```python
from build123d import *

# Parameters (mm, degrees)
BOSS_EXTRUDE1_DEPTH       = 51
BOSS_EXTRUDE3_DEPTH       = 51
SKETCH2_5_R               = 4.5
BOSS_EXTRUDE4_DEPTH       = 9
CUT_EXTRUDE2_REACH        = 105.296
SKETCH3_R                 = 4.5
CUT_EXTRUDE3_REACH        = 105.296
BOSS_EXTRUDE5_REACH       = 105.296
SKETCH4_R                 = 8
F_6_0MM_DOWEL_HOLE1_D     = 6
F_6_0MM_DOWEL_HOLE1_DEPTH = 13
F_6_0MM_DOWEL_HOLE1_TIP   = 1.802581857


with BuildPart() as part:
    # Sketch2 → Boss-Extrude1 (new body)
    with BuildSketch(Plane.XY):
        with BuildLine():
            ThreePointArc((40, 0), (39.453405592, 6.590052141), (37.828560639, 13))
            ThreePointArc((37.828560639, 13), (0, 40), (-37.828560639, 13))
            ThreePointArc((-37.828560639, 13), (-39.453405592, 6.590052141), (-40, 0))
            Line((-40, 0), (-26.965, 0))
            ThreePointArc((-26.965, 0), (0, 26.965), (26.965, 0))
            Line((26.965, 0), (40, 0))
        make_face()
    extrude(amount=BOSS_EXTRUDE1_DEPTH)

    # Sketch2<4> → Boss-Extrude3 (add)
    with BuildSketch(Plane.XY):
        with BuildLine():
            ThreePointArc((-40, 0), (-39.453405592, 6.590052141), (-37.828560639, 13))
            Line((-37.828560639, 13), (-63.686733312, 13))
            Line((-63.686733312, 13), (-65, 13))
            Line((-65, 13), (-65, 0))
            Line((-65, 0), (-40, 0))
        make_face()
        with BuildLine():
            Line((63.686733312, 13), (37.828560639, 13))
            ThreePointArc((37.828560639, 13), (39.453405592, 6.590052141), (40, 0))
            Line((40, 0), (65, 0))
            Line((65, 0), (65, 13))
            Line((65, 13), (63.686733312, 13))
        make_face()
    extrude(amount=BOSS_EXTRUDE3_DEPTH)

    # Sketch2<5> → Boss-Extrude4 (add)
    with BuildSketch(Plane.XY):
        with BuildLine():
            ThreePointArc((-37.828560639, 13), (0, 40), (37.828560639, 13))
            Line((37.828560639, 13), (63.686733312, 13))
            ThreePointArc((63.686733312, 13), (48.281028578, 43.519447141), (19.519221296, 62))
            Line((19.519221296, 62), (-19.519221296, 62))
            ThreePointArc((-19.519221296, 62), (-48.281028578, 43.519447141), (-63.686733312, 13))
            Line((-63.686733312, 13), (-37.828560639, 13))
        make_face()
        with Locations((-41, 32)):
            Circle(SKETCH2_5_R, mode=Mode.SUBTRACT)
        with Locations((41, 32)):
            Circle(SKETCH2_5_R, mode=Mode.SUBTRACT)
    extrude(amount=BOSS_EXTRUDE4_DEPTH)

    # Sketch3 → Cut-Extrude2 (cut, up to next)
    with BuildSketch(Plane(origin=(0, 0, 0), x_dir=(1, 0, 0), z_dir=(0, 1, 0)), mode=Mode.PRIVATE) as cut_extrude2_sk1:
        with BuildLine():
            Line((37.828560639, -51), (65, -51))
            Line((65, -51), (65, -21))
            ThreePointArc((65, -21), (63.859756378, -26.324112946), (60.639049437, -30.714258841))
            Line((60.639049437, -30.714258841), (37.828560639, -51))
        make_face()
    cut_extrude2_tool1 = extrude(cut_extrude2_sk1.sketch, amount=CUT_EXTRUDE2_REACH, mode=Mode.PRIVATE) & part.part
    # Sketch3 → Cut-Extrude2 (cut, up to next)
    with BuildSketch(Plane(origin=(0, 0, 0), x_dir=(1, 0, 0), z_dir=(0, 1, 0)), mode=Mode.PRIVATE) as cut_extrude2_sk2:
        with Locations(Location((52, -21, 0), (0, 0, 270))):
            Circle(SKETCH3_R)
    cut_extrude2_tool2 = extrude(cut_extrude2_sk2.sketch, amount=CUT_EXTRUDE2_REACH, mode=Mode.PRIVATE) & part.part
    # Sketch3 → Cut-Extrude2 (cut, up to next)
    with BuildSketch(Plane(origin=(0, 0, 0), x_dir=(1, 0, 0), z_dir=(0, 1, 0)), mode=Mode.PRIVATE) as cut_extrude2_sk3:
        with Locations(Location((-52, -21, 0), (0, 0, 270))):
            Circle(SKETCH3_R)
    cut_extrude2_tool3 = extrude(cut_extrude2_sk3.sketch, amount=CUT_EXTRUDE2_REACH, mode=Mode.PRIVATE) & part.part
    add(cut_extrude2_tool1.solids().sort_by_distance((56.054542, 0, 42.719243))[0], mode=Mode.SUBTRACT)
    add(cut_extrude2_tool2.solids().sort_by_distance((52, 0, 21))[0], mode=Mode.SUBTRACT)
    add(cut_extrude2_tool3.solids().sort_by_distance((-52, 0, 21))[0], mode=Mode.SUBTRACT)

    # Sketch3<4> → Cut-Extrude3 (cut, up to next)
    with BuildSketch(Plane(origin=(0, 0, 0), x_dir=(1, 0, 0), z_dir=(0, 1, 0)), mode=Mode.PRIVATE) as cut_extrude3_sk1:
        with BuildLine():
            Line((-65, -51), (-37.828560639, -51))
            Line((-37.828560639, -51), (-60.639049437, -30.714258841))
            ThreePointArc((-60.639049437, -30.714258841), (-63.859756378, -26.324112946), (-65, -21))
            Line((-65, -21), (-65, -51))
        make_face()
    cut_extrude3_tool1 = extrude(cut_extrude3_sk1.sketch, amount=CUT_EXTRUDE3_REACH, mode=Mode.PRIVATE) & part.part
    add(cut_extrude3_tool1.solids().sort_by_distance((-56.054542, 0, 42.719243))[0], mode=Mode.SUBTRACT)

    # Boss-Extrude5: up to this face of the body (flat: up to its plane)
    boss_extrude5_end = Plane(part.part.faces().sort_by_distance((-47.267324257, 42.605716574, 9))[0])
    # Sketch4 → Boss-Extrude5 (add, up to the picked face)
    with BuildSketch(Plane.XY.offset(51), mode=Mode.PRIVATE) as boss_extrude5_sk1:
        with Locations((-36, 14)):
            Circle(SKETCH4_R)
    boss_extrude5_tool1 = split(extrude(boss_extrude5_sk1.sketch, amount=-BOSS_EXTRUDE5_REACH, mode=Mode.PRIVATE), bisect_by=boss_extrude5_end, keep=Keep.BOTH, mode=Mode.PRIVATE)
    add(boss_extrude5_tool1.solids().sort_by(Axis((-36, 14, 51), (0, 0, -1)))[0])

    # Ø6.0mm Dowel Hole1
    with Locations(Plane(origin=(-38.545011934, 12.938196737, 51), x_dir=(1, 0, 0), z_dir=(0, 0, 1))):
        with Locations((0, 0)):
            Hole(F_6_0MM_DOWEL_HOLE1_D / 2, depth=F_6_0MM_DOWEL_HOLE1_DEPTH)
            with Locations((0, 0, -(F_6_0MM_DOWEL_HOLE1_DEPTH + F_6_0MM_DOWEL_HOLE1_TIP / 2))):  # 118° drill point
                Cone(0, F_6_0MM_DOWEL_HOLE1_D / 2, F_6_0MM_DOWEL_HOLE1_TIP, mode=Mode.SUBTRACT)


solid = part.part
```
The model under review builds one solid part; all positions refer to its coordinate system, in mm. A direction names the side the tool comes from. Round coordinates to 2 decimals unless told otherwise and drop trailing zeros. Loops run counter-clockwise (first coordinate to the right, second up) from the corner with the lowest first, then second, coordinate; pieces in that order, holes last. Notation, with made-up numbers: M -4.5,68 L 14.5,68 A12 cw 14.5,84 Z; hole C 34,-28 d11. An arc over 180 degrees is marked long. Put each result on its own line as item: value.
Q1. Consider section D-D, the plane y = 56. Give the boundary of the cut face in (x, z).
Result set:
outline: M -33,0 L 33,0 L 33,9 L -33,9 Z
Q2. Consider section C-C, the plane x = 0. Give the boundary of the cut face in (y, z) (3 decimals).
Result set:
outline: M 26.965,0 L 62,0 L 62,9 L 40,9 L 40,51 L 26.965,51 Z
Q3. To check wall thickness, follow L1, parallel to X at y = 9.5, z = 21; L2, parallel to Y at x = 44, z = 24; L3, parallel to Y at x = 41, z = 3. State the ranges of each line that lie inside material, in increasing order.
Result set:
L1: x = -65 to -56.5, -47.5 to -25.24, 25.24 to 47.5, 56.5 to 65
L2: y = 0 to 13
L3: y = 0 to 27.5, 36.5 to 50.44
Q4. Consider section A-A, the plane x = -52. Give the boundary of the cut face in (y, z), then the cut area to 3 significant figures.
Result set:
outline: M 0,0 L 39,0 L 39,9 L 13,9 L 13,16.5 L 0,16.5 Z; M 0,25.5 L 13,25.5 L 13,38.4 L 0,38.4 Z
area: 616 mm²
Q5. Consider section B-B, the plane z = 23.5. Give the boundary of the cut face in (x, y) (3 decimals).
Result set:
outline: M -64.757,0 L -55.742,0 L -55.742,13 L -64.757,13 Z; M -48.258,0 L -26.965,0 A26.965 cw 26.965,0 L 48.258,0 L 48.258,13 L 37.829,13 A40 ccw -33.639,21.644 A8 ccw -43.937,13 L -48.258,13 Z; M 55.742,0 L 64.757,0 L 64.757,13 L 55.742,13 Z
Q6. For pin 1 (8 mm diameter, centred on x = -2, z = 32, fed in from +Y); pin 2 (7 mm diameter, centred on x = -41, y = 32, fed in from -Z); pin 3 (24.5 mm diameter, centred on x = -31, y = 47, fed in from +Z); pin 4 (8 mm diameter, centred on y = 31.5, z = 31, fed in from -X), all flat-tipped, find the tip position at first contact; note any pin that passes through.
Result set:
pin 1: stops at y = 40
pin 2: passes through
pin 3: stops at z = 9
pin 4: stops at x = -29.05
Q7. Machinability: for faces 1 (the cylindrical face through (-35.548, 13.07, 44.409)), 2 (the cylindrical face through (47.61, 6.41, 20.02)), 3 (the cylindrical face through (5.42, 39.63, 29.71)), which of the approach directions +Z, -Z, +X, -X, +Y, -Y give a long, thin tool a straight path to every point of the face, cutting with its end or side? Answer none if there is none.
Result set:
face 1: +Z
face 2: +Y, -Y
face 3: +Z, +Y
Q8. Mouldability with a two-part tool opening along Y and no side actions: class faces 4 (the conical face through (-38.96, 12.62, 36.51)), 5 (the flat face through (41, 0, 19)), 6 (the flat face through (0, 62, 4)), 7 (the flat face through (-65, 7, 10)) as released by +Y, released by -Y, zero draft, split by the parting line, or undercut.
Result set:
face 4: undercut
face 5: released by -Y
face 6: released by +Y
face 7: zero draft
